```python
from build123d import *

# Parameters (mm, degrees)
F0_R            = 165.5
F0_R_2          = 147
F1_DEPTH        = 3
F2_R            = 3
F3_DEPTH        = 25
F3_COPIES_COUNT = 11


# Not quite as in the source:
# - a pattern or mirror of a feature is missing from the dataset's text; its kind, count and spacing are read off the source's solid


with BuildPart() as f1:
    # F0 (on Front) → F1 (new body)
    with BuildSketch(Plane.XZ):
        Circle(F0_R)
        Circle(F0_R_2, mode=Mode.SUBTRACT)
    extrude(amount=F1_DEPTH)

    # F2 (on face) → F3 (cut)
    with BuildSketch(Plane.XZ.offset(3)):
        with Locations((0, 156.4114242792)):
            Circle(F2_R)
    f3 = extrude(amount=-F3_DEPTH, mode=Mode.SUBTRACT)

    # F3_copies: F3 ×11 about axis
    f3_copies_axis = Axis((0, 0, 0), (0, 1, 0))
    for i in range(1, F3_COPIES_COUNT):
        add(f3.rotate(f3_copies_axis, i * 360 / F3_COPIES_COUNT), mode=Mode.SUBTRACT)


solid = f1.part
```
Geometry: final body of the model. Coordinates: model frame, mm. Round coordinates to 2 decimals unless told otherwise and drop trailing zeros. Loops run counter-clockwise (first coordinate to the right, second up) from the corner with the lowest first, then second, coordinate; pieces in that order, holes last. Notation, with made-up numbers: (-35, 15) -> (17, 15) arc R7 ccw to (17, 24) -> close; hole circle Ø10 at (55.5, 10). An arc over 180 degrees is marked (long way). Use one line per item in the form item = value.
Item 1: Cut plane B-B on x = -77.5. Output: boundary loops of the cut face in (y, z).
Evaluation:
outline = (-3, -146.23) -> (0, -146.23) -> (0, -124.91) -> (-3, -124.91) -> close; (-3, 124.91) -> (0, 124.91) -> (0, 146.23) -> (-3, 146.23) -> close
Item 2: Cut plane C-C on y = -1.15. Give the number of separate pieces and of enclosed holes in the cut face, then the cut area to 3 significant figures.
Evaluation:
separate_pieces = 1
enclosed_holes = 12
area = 17,900 mm2
Item 3: Draft query along X for faces 1 (the cylindrical face through (-31.867, -1.479, -143.504)), 2 (the cylindrical face through (-35.877, -1.479, -161.564)), 3 (the flat face through (-1, -3, 148)). Return one class per face: released by +X, released by -X, zero draft, split by the parting line, or undercut.
Evaluation:
face_1 = undercut
face_2 = split by the parting line
face_3 = zero draft
Item 4: Material intervals for probe 1 along X at (y, z) = (-1.2, 3); probe 2 along Z at (x, y) = (-2.5, -1.15); probe 3 along Z at (x, y) = (-84.5, -1.05), sorted ascending.
Evaluation:
probe_1 = -165.47 to -146.97, 146.97 to 165.47
probe_2 = -165.48 to -146.98, 146.98 to 154.75, 158.07 to 165.48
probe_3 = -142.3 to -120.29, 120.29 to 128.58, 134.58 to 142.3
Item 5: Contact query for flat-ended pins moving along their axis: pin 1 Ø1 at (y, z) = (-0.5, 49) entering from -X; pin 2 Ø1.5 at (y, z) = (-1.5, 10.5) entering from -X; pin 3 Ø1.5 at (y, z) = (-0.5, 55) entering from +X. Output: stop coordinate, or through.
Evaluation:
pin_1 = -158.23
pin_2 = -165.21
pin_3 = 156.36
Item 6: Cut plane A-A on z = 0. Output: boundary loops of the cut face in (x, y).
Evaluation:
outline = (-165.5, -3) -> (-147, -3) -> (-147, 0) -> (-165.5, 0) -> close; (147, -3) -> (165.5, -3) -> (165.5, 0) -> (147, 0) -> close
